Part model, mm, in its own coordinate system. A direction names the side the tool comes from. Round coordinates to 2 decimals unless told otherwise and drop trailing zeros. Put each result on its own line as item: value. Start each with the question number.
```python
from build123d import *

# Parameters (mm, degrees)
F0_W     = 350
F0_H     = 140
F1_DEPTH = 20
F9_DEPTH = 6.2
F11_D    = 6


with BuildPart() as f1:
    # F0 (on Top) → F1 (new body)
    with BuildSketch(Plane.XY):
        with Locations((175, 70)):
            Rectangle(F0_W, F0_H)
    extrude(amount=-F1_DEPTH)

    # F4 (on plane+point) → F7 section 0
    with BuildSketch(Plane.XZ.offset(-35)):
        with BuildLine():
            Line((128, 0), (20, 0))
            Line((20, 0), (20, -0.8))
            add(Edge.make_bspline(
                [(20, -0.8), (33.539250493, -13.4811280295), (116.6631821028, -3.1675355221), (128, -0.8)],
                knots=[0, 0, 0, 0, 108, 108, 108, 108], degree=3))
            Line((128, -0.8), (128, 0))
        make_face()
    # F6 (on plane+point) → F7 section 1
    with BuildSketch(Plane.XZ.offset(-120)):
        with BuildLine():
            Line((155, 0), (75, 0))
            Line((75, 0), (75, -0.8))
            add(Edge.make_bspline(
                [(75, -0.8), (83.8186404567, -8.6791180032), (137.2789575916, -3.563235641), (155, -0.8)],
                knots=[0, 0, 0, 0, 80, 80, 80, 80], degree=3))
            Line((155, -0.8), (155, 0))
        make_face()
    loft(mode=Mode.SUBTRACT)

    # F8 (on Top) → F9 (cut)
    with BuildSketch(Plane.XY):
        with BuildLine():
            Line((50, 35), (30, 35))
            Line((30, 35), (30, 22))
            ThreePointArc((30, 22), (30.5857864376, 20.5857864376), (32, 20))
            Line((32, 20), (48, 20))
            ThreePointArc((48, 20), (49.4142135624, 20.5857864376), (50, 22))
            Line((50, 22), (50, 35))
        make_face()
        with BuildLine():
            Line((103, 35), (83, 35))
            Line((83, 35), (83, 22))
            ThreePointArc((83, 22), (83.5857864376, 20.5857864376), (85, 20))
            Line((85, 20), (101, 20))
            ThreePointArc((101, 20), (102.4142135624, 20.5857864376), (103, 22))
            Line((103, 22), (103, 35))
        make_face()
    extrude(amount=-F9_DEPTH, mode=Mode.SUBTRACT)

    # F11 (through all)
    with Locations(Plane.XY):
        with Locations((66.5, 16), (145, 124)):
            Hole(F11_D / 2)


solid = f1.part
```
1. Drop flat-ended pins along their axis: pin 1 (3 mm diameter, centred on y = 29.5, z = -4, fed in from -X); pin 2 (4.5 mm diameter, centred on x = 93, y = 28, fed in from +Z). Give the stop position or say it passes through.
2. Wall check: L1, parallel to Y at x = 66.5, z = -16; L2, parallel to Y at x = 145, z = -12.75; L3, parallel to Z at x = 139, y = 76. Give the ranges that are in metal, low to high.
3. Which spindle directions (+Z, -Z, +X, -X, +Y, -Y) get a long thin tool onto all of the face, cutting with end or side? Do faces 1 (the flat face through (83, 29, -3)), 2 (the flat face through (173, 140, -10)). Say none if no direction does.
4. Mould opens along X. For faces 3 (the flat face through (66, 35, -4)), 4 (the flat face through (30, 29, -3)), 5 (the flat face through (0, 69, -10)), 6 (the flat face through (173, 71, 0)) say: released by +X, released by -X, zero draft, split by the parting line, or undercut.
Results list:
1. pin 1: stops at x = 0
1. pin 2: stops at z = -6.2
2. L1: y = 0 to 13, 19 to 140
2. L2: y = 0 to 121, 127 to 140
2. L3: z = -20 to -1.14
3. face 1: +Z
3. face 2: +Z, -Z, +X, -X, +Y
4. face 3: undercut
4. face 4: undercut
4. face 5: released by -X
4. face 6: zero draft
